Geometry check sheet. Reference: drawing and pictorial views, mm from the part's lowest x, y, z. A direction names the side the tool comes from. Round coordinates to 2 decimals unless told otherwise and drop trailing zeros. Order: outer loops, then holes, each group sorted by start corner. A loop starts at its lowest first (then second) coordinate and runs counter-clockwise, first axis right, second up.
Q1. Cross-section at D-D on x = 2. Record the cut outline in (y, z), then the cut area to 3 significant figures.
Q2. Cross-section at C-C on x = 5.4. Record the cut outline in (y, z), then the cut area to 3 significant figures.
Q3. Scan lines: probe 1 along Y at (x, z) = (2.6, 4); probe 2 along Y at (x, z) = (4.85, 4); probe 3 along X at (y, z) = (1.25, 2.5). Record each from-to range of solid material in increasing order.
Q4. Set-up check for the marked faces 1 and 2: record each of +Z, -Z, +X, -X, +Y, -Y from which the full face is reachable in a straight line by a thin tool's end or side.
Q5. Mould release check, pull along Y, two halves, no side actions. Record for the marked faces 3, 4 and 5: +Y half, -Y half, draft (parallel to the pull), parting line (faces both ways), or undercut.
Q6. Depth check by flat-ended pin: P1, Ø1.5, axis at x = 2, y = 1.5, coming from the -Z side; P2, Ø1, axis at x = 4.5, z = 6, coming from the +Y side. Enter the tip coordinate at first touch or a pass-through.
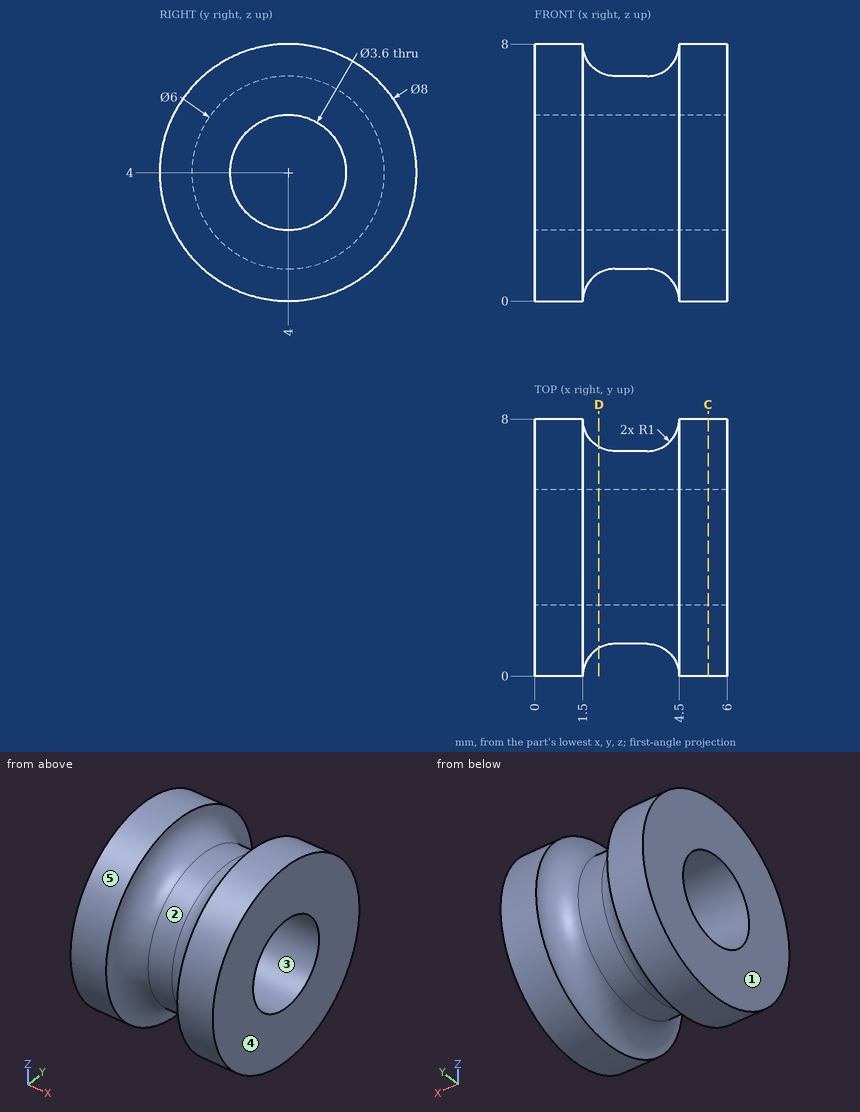
Results found:
1. outline: circle Ø6.27 at (4, 4); hole circle Ø3.6 at (4, 4)
1. area: 20.7 mm2
2. outline: circle Ø8 at (4, 4); hole circle Ø3.6 at (4, 4)
2. area: 40.1 mm2
3. probe 1: y = 1 to 2.2, 5.8 to 7
3. probe 2: y = 0 to 2.2, 5.8 to 8
3. probe 3: x = 0 to 2, 4 to 6
4. face 1: +Z, -Z, -X, +Y, -Y
4. face 2: none
5. face 3: undercut
5. face 4: draft
5. face 5: parting line
6. P1: stops at z = 0.5
6. P2: stops at y = 7.71
